```python
from build123d import *

# Parameters (mm, degrees)
SKETCH1_W           = 9.525
SKETCH1_H           = 76.2
BOSS_EXTRUDE1_DEPTH = 31.75
SKETCH2_R           = 1.778
CUT_EXTRUDE1_DEPTH  = 10.525
SKETCH3_R           = 1.7272
CUT_EXTRUDE2_DEPTH  = 19.05


with BuildPart() as part:
    # Sketch1 → Boss-Extrude1 (new body)
    with BuildSketch(Plane.XY):
        with Locations((4.7625, 38.1)):
            Rectangle(SKETCH1_W, SKETCH1_H)
    extrude(amount=BOSS_EXTRUDE1_DEPTH)

    # Sketch2 → Cut-Extrude1 (cut, through all)
    with BuildSketch(Plane.ZY):
        with Locations((5.9182, 57.15)):
            Circle(SKETCH2_R)
        with Locations((5.9182, 19.05)):
            Circle(SKETCH2_R)
    extrude(amount=-CUT_EXTRUDE1_DEPTH, mode=Mode.SUBTRACT)

    # Sketch3 → Cut-Extrude2 (cut)
    with BuildSketch(Plane.XZ):
        with Locations((4.7625, 25.4)):
            Circle(SKETCH3_R)
        with Locations((4.7625, 12.7)):
            Circle(SKETCH3_R)
    extrude(amount=-CUT_EXTRUDE2_DEPTH, mode=Mode.SUBTRACT)


solid = part.part
```
The listing builds one solid part. Answer for the finished solid, in the listing's coordinates (mm). A direction names the side the tool comes from. Give positions to 0.01 mm unless a question says otherwise; leave off trailing zeros. Loops run counter-clockwise (first coordinate to the right, second up) from the corner with the lowest first, then second, coordinate; pieces in that order, holes last. Notation, with made-up numbers: (-30, 42) - (17, 42) arc R17 cw to (17, 59) - close; hole circle Ø9 at (-21.75, 59.25). An arc over 180 degrees is marked (long way). Return JSON: item names as keys, results as strings. Group by question number.
1. Straight lines are drawn through the part: line 1 (Z direction, x = 3.5, y = 14); line 2 (X direction, y = 9, z = 12) (1 decimal); line 3 (Y direction, x = 2, z = 4.5). For each, find the intervals that lie inside material, in ascending order. Write a range as [from, to].
2. Which of the six approach directions +Z, -Z, +X, -X, +Y, -Y give full straight-line access (tool end or side, diameter ignored) to faces 5 (the cylindrical face through (5.56, 9.39, 11.17)), 6 (the flat face through (5, 76.2, 16))?
3. Find section A-A (z = 25.4). Write down the section's boundary in (x, y) (3 decimals), then the cut area to 3 significant figures.
4. Determine the mould class of faces 1 (the cylindrical face through (4.696, 58.913, 5.687)), 2 (the flat face through (9.525, 38, 16)), 3 (the flat face through (5, 0, 16)), 4 (the cylindrical face through (4.696, 20.813, 5.687)) for opening direction Y: pulls with the +Y half, pulls with the -Y half, needs draft (parallel to the pull), parting line crosses it, or undercut.
5. Given pin 1 Ø1.7 at (x, z) = (5, 12) entering from -Y; pin 2 Ø3 at (y, z) = (19.05, 5.92) entering from -X, each flat-ended and moving along its own axis, determine where each tip first touches the part or whether it passes through.
6. Find section B-B (x = 4.5). Write down the section's boundary in (y, z).
Verdict:
{
 "1": {"line 1": "z = [0, 11.52], [13.88, 24.22], [26.58, 31.75]", "line 2": "x = [0, 3.2], [6.3, 9.5]", "line 3": "y = [0, 17.98], [20.12, 56.08], [58.22, 76.2]"},
 "2": {"face 5": "-Y", "face 6": "+Z, -Z, +X, -X, +Y"},
 "3": {"outline": "(0, 0) - (3.035, 0) - (3.035, 19.05) - (6.49, 19.05) - (6.49, 0) - (9.525, 0) - (9.525, 76.2) - (0, 76.2) - close", "area": "660 mm^2"},
 "4": {"face 1": "undercut", "face 2": "needs draft", "face 3": "pulls with the -Y half", "face 4": "undercut"},
 "5": {"pin 1": "stops at y = 19.05", "pin 2": "passes through"},
 "6": {"outline": "(0, 0) - (76.2, 0) - (76.2, 31.75) - (0, 31.75) - (0, 27.11) - (19.05, 27.11) - (19.05, 23.69) - (0, 23.69) - (0, 14.41) - (19.05, 14.41) - (19.05, 10.99) - (0, 10.99) - close; hole circle Ø3.56 at (19.05, 5.92); hole circle Ø3.56 at (57.15, 5.92)"}
}
